Read the model definition and answer for the solid it produces. Units are mm, in the model's axes. Face numbers are marked on the shaded views. A direction names the side the tool comes from. Give positions to 0.01 mm unless a question says otherwise; leave off trailing zeros. Order: outer loops, then holes, each group sorted by start corner. A loop starts at its lowest first (then second) coordinate and runs counter-clockwise, first axis right, second up.
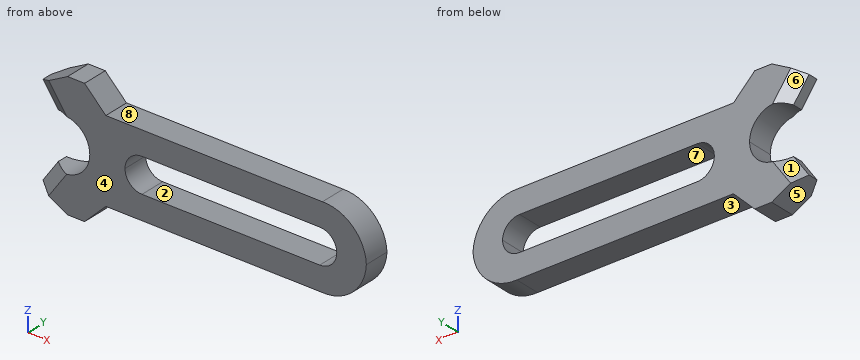
```python
from build123d import *

# Parameters (mm, degrees)
BOSS_EXTRUDE1_DEPTH = 3.8227
CHAMFER1_SIZE       = 1.17
CHAMFER1_SIZE2      = 2.026499445


with BuildPart() as part:
    # Sketch1 → Boss-Extrude1 (new body)
    with BuildSketch(Plane(origin=(0, 0, 0), x_dir=(1, 0, 0), z_dir=(0, 1, 0))):
        with BuildLine():
            ThreePointArc((13.950769004, 0.075877145), (11.919896105, 4.457709898), (7.394873867, 6.145630734))
            Line((7.394873867, 6.145630734), (-24.953822463, 6.145630734))
            Line((-24.953822463, 6.145630734), (-28.128822463, 9.320630734))
            Line((-28.128822463, 9.320630734), (-30.668822463, 9.320630734))
            Line((-30.668822463, 9.320630734), (-35.284454716, 6.802487588))
            Line((-35.284454716, 6.802487588), (-32.99014897, 3.525879411))
            ThreePointArc((-32.99014897, 3.525879411), (-29.206377785, 3.379332749), (-27.355545164, 0.075877145))
            Line((-27.355545164, 0.075877145), (-22.092646818, 0.075877145))
            ThreePointArc((-22.092646818, 0.075877145), (-21.348698042, 1.87192837), (-19.552646818, 2.615877145))
            Line((-19.552646818, 2.615877145), (6.926853182, 2.615877145))
            Line((6.926853182, 2.615877145), (6.990353182, 2.615877145))
            ThreePointArc((6.990353182, 2.615877145), (8.786404406, 1.87192837), (9.530353182, 0.075877145))
            Line((9.530353182, 0.075877145), (13.950769004, 0.075877145))
        make_face()
    extrude(amount=BOSS_EXTRUDE1_DEPTH)

    # Chamfer1
    chamfer1_edges = [part.edges().sort_by_distance(p)[0] for p in [
        (-34.137301843, 0, -5.1641835),
        (-34.137301843, 3.8227, -5.1641835),
    ]]
    chamfer1_side = [part.faces().sort_by_distance(p)[0] for p in [
        (-34.137301843, 1.91135, -5.1641835),
    ]]
    chamfer(chamfer1_edges, length=CHAMFER1_SIZE, length2=CHAMFER1_SIZE2, reference=chamfer1_side[0])

    # Mirror1: part across plane


with BuildPart() as part_1:
    add(part.part)
    add(part.part.mirror(Plane(origin=(0, 3.8227, -0.075877145), x_dir=(1, 0, 0), z_dir=(0, 0, 1))))


solid = part_1.part
```
1) The part is cut by section C-C on z = -1. Determine the outline of the cut face in (x, y), and give its area (3 significant figures).
Final values:
outline: (-27.47, 0) - (-21.92, 0) - (-21.92, 3.82) - (-27.47, 3.82) - close; (9.36, 0) - (13.84, 0) - (13.84, 3.82) - (9.36, 3.82) - close
area: 38.4 mm2
2) The part is cut by section B-B on x = 3. Determine the outline of the cut face in (y, z).
Final values:
outline: (0, -6.15) - (3.82, -6.15) - (3.82, -2.62) - (0, -2.62) - close; (0, 2.46) - (3.82, 2.46) - (3.82, 5.99) - (0, 5.99) - close
3) The part is cut by section D-D on x = -24. Determine the outline of the cut face in (y, z).
Final values:
outline: (0, -6.15) - (3.82, -6.15) - (3.82, 5.99) - (0, 5.99) - close
4) For a pull along Z with two mould halves and no side action, classify the marked faces 5, 6, 7 and 8 as released by +Z, released by -Z, zero draft, split by the parting line, or undercut.
Final values:
face 5: released by -Z
face 6: undercut
face 7: undercut
face 8: released by +Z
5) Given pin 1 (2 mm diameter, centred on y = 2, z = 6.5, fed in from -X); pin 2 (1.9 mm diameter, centred on x = -12, y = 1.5, fed in from +Z); pin 3 (1.9 mm diameter, centred on x = -5, y = 2.5, fed in from -Z); pin 4 (2 mm diameter, centred on y = 2.5, z = 4, fed in from -X), each flat-ended and moving along its own axis, determine where each tip first touches the part or whether it passes through.
Final values:
pin 1: stops at x = -35.28
pin 2: stops at z = 5.99
pin 3: stops at z = -6.15
pin 4: stops at x = -34.13
6) A tool of negligible diameter and unlimited length cuts with its end or side. For the marked faces 1, 2, 3 and 4, from which of +Z, -Z, +X, -X, +Y, -Y can it reach the whole face along a straight path? Write none if from no direction.
Final values:
face 1: -X, +Y
face 2: +Y, -Y
face 3: -Z, +X, +Y, -Y
face 4: +Z, -Z, +X, -X, -Y
7) The part is cut by section A-A on y = 1.7. Determine the outline of the cut face in (x, z).
Final values:
outline: (-35.28, -6.8) - (-30.67, -9.32) - (-28.13, -9.32) - (-24.95, -6.15) - (7.39, -6.15) arc R6.35 ccw to (13.95, -0.08) arc R6.35 ccw to (7.39, 5.99) - (-24.95, 5.99) - (-28.13, 9.17) - (-30.67, 9.17) - (-35.28, 6.65) - (-32.99, 3.37) arc R3.87 cw (long way) to (-32.99, -3.53) - close; hole (-19.55, -2.62) - (6.99, -2.62) arc R2.54 ccw to (6.99, 2.46) - (-19.55, 2.46) arc R2.54 ccw to start
8) Consider L1, parallel to Z at x = 1, y = 2.4; L2, parallel to Z at x = -21, y = 1.65; L3, parallel to X at y = 0.3, z = -2. Determine where each line is inside the solid, lowest interval first.
Final values:
L1: z = -6.15 to -2.62, 2.46 to 5.99
L2: z = -6.15 to -2.16, 2.01 to 5.99
L3: x = -27.87 to -21.21, 8.65 to 13.56
